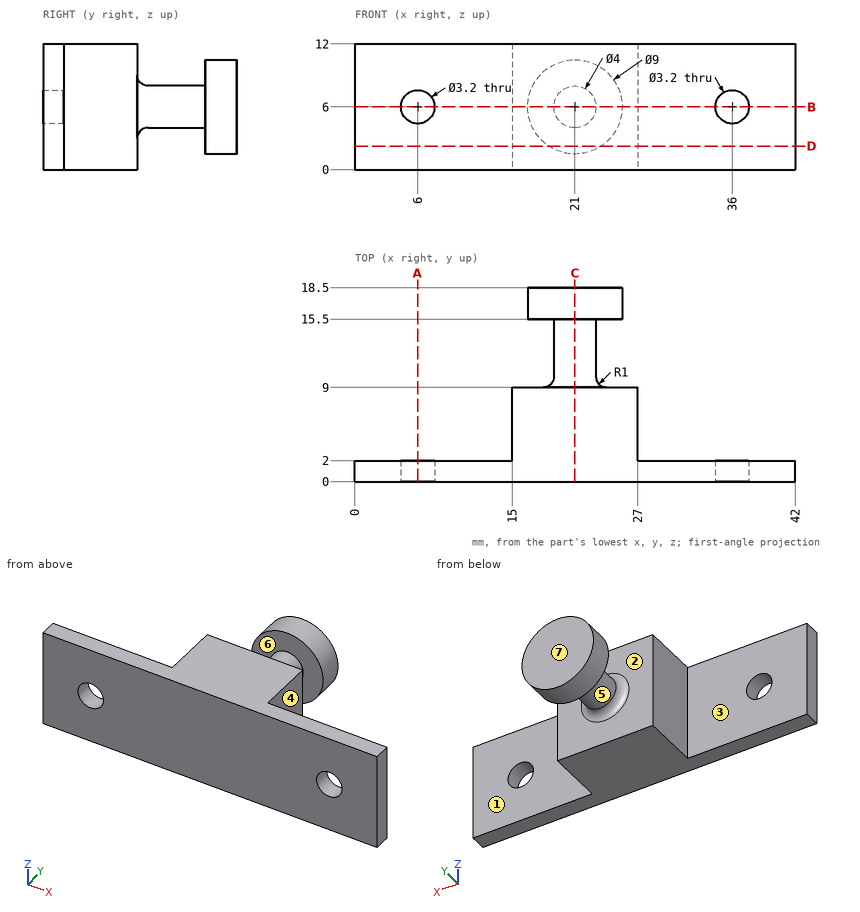
Geometry: see drawing. Coordinates: mm, zero at the bounding-box minimum. A direction names the side the tool comes from. Give positions to 0.01 mm unless a question says otherwise; leave off trailing zeros. Order: outer loops, then holes, each group sorted by start corner. A loop starts at its lowest first (then second) coordinate and runs counter-clockwise, first axis right, second up.
Q1. Ray query, probe 1 along X at (y, z) = (0.9, 6); probe 2 along X at (y, z) = (6, 8.5); probe 3 along Y at (x, z) = (30, 2.25). Return the intervals inside material, ascending.
Checked values:
probe 1: x = 0 to 4.4, 7.6 to 34.4, 37.6 to 42
probe 2: x = 15 to 27
probe 3: y = 0 to 2
Q2. Draft query along Y for the marked faces 4, 5, 6 and 7. Return one class per face: +Y half, -Y half, draft (parallel to the pull), parting line (faces both ways), or undercut.
Checked values:
face 4: draft
face 5: undercut
face 6: undercut
face 7: +Y half
Q3. Set-up query: the marked faces 1, 2 and 3. Return all of +Z, -Z, +X, -X, +Y, -Y with unobstructed straight access to the full face (end or side cutting, diameter ignored); none if empty.
Checked values:
face 1: +Z, -Z, +X, +Y
face 2: none
face 3: +Z, -Z, -X, +Y
Q4. Contact query for flat-ended pins moving along their axis: pin 1 Ø1.5 at (x, y) = (14.5, 10.5) entering from +Z; pin 2 Ø1 at (x, z) = (15, 9) entering from +Y; pin 3 Ø1 at (y, z) = (8, 7.5) entering from +X; pin 4 Ø3.5 at (x, z) = (6, 6) entering from +Y. Output: stop coordinate, or through.
Checked values:
pin 1: passes through
pin 2: stops at y = 9
pin 3: stops at x = 27
pin 4: stops at y = 2
Q5. Section D-D on z = 2.25. Output: boundary loops of the cut face in (x, y), and give its area (3 significant figures).
Checked values:
outline: (0, 0) - (42, 0) - (42, 2) - (27, 2) - (27, 9) - (15, 9) - (15, 2) - (0, 2) - close; (18.51, 15.5) - (23.49, 15.5) - (23.49, 18.5) - (18.51, 18.5) - close
area: 183 mm2
Q6. Section C-C on x = 21. Output: boundary loops of the cut face in (y, z).
Checked values:
outline: (0, 0) - (9, 0) - (9, 3) arc R1 cw to (10, 4) - (15.5, 4) - (15.5, 1.5) - (18.5, 1.5) - (18.5, 10.5) - (15.5, 10.5) - (15.5, 8) - (10, 8) arc R1 cw to (9, 9) - (9, 12) - (0, 12) - close
Q7. Section A-A on x = 6. Output: boundary loops of the cut face in (y, z).
Checked values:
outline: (0, 0) - (2, 0) - (2, 4.4) - (0, 4.4) - close; (0, 7.6) - (2, 7.6) - (2, 12) - (0, 12) - close
Q8. Section B-B on z = 6. Output: boundary loops of the cut face in (x, y).
Checked values:
outline: (0, 0) - (4.4, 0) - (4.4, 2) - (0, 2) - close; (7.6, 0) - (34.4, 0) - (34.4, 2) - (27, 2) - (27, 9) - (24, 9) arc R1 cw to (23, 10) - (23, 15.5) - (25.5, 15.5) - (25.5, 18.5) - (16.5, 18.5) - (16.5, 15.5) - (19, 15.5) - (19, 10) arc R1 cw to (18, 9) - (15, 9) - (15, 2) - (7.6, 2) - close; (37.6, 0) - (42, 0) - (42, 2) - (37.6, 2) - close
